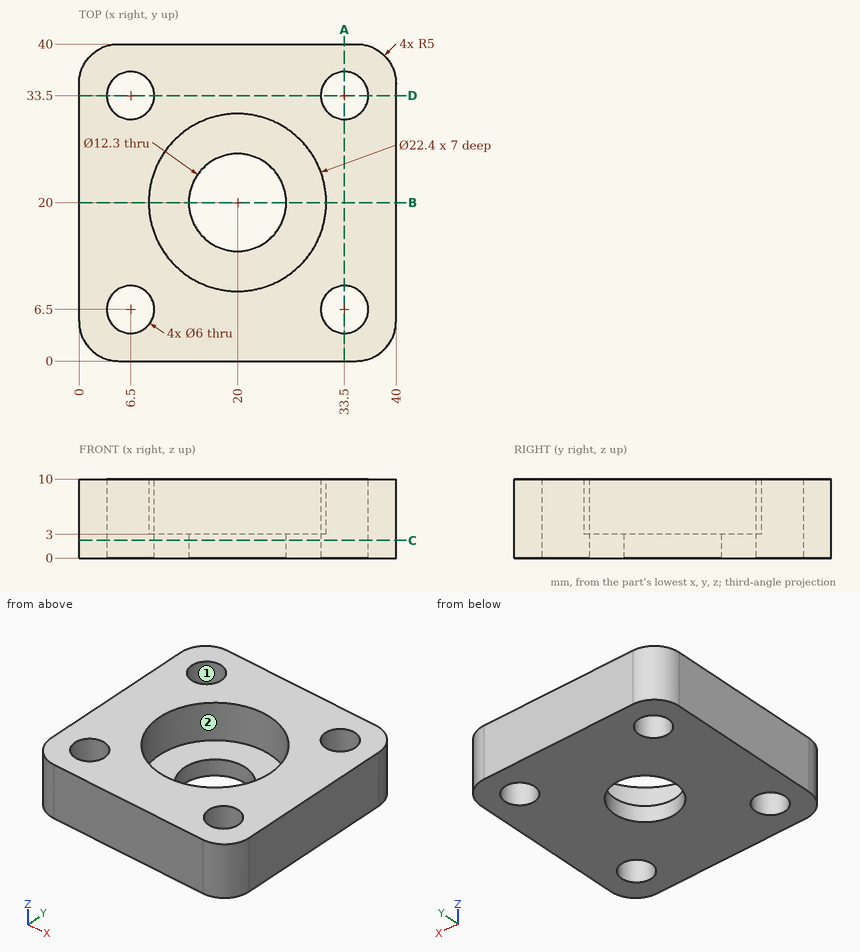
Drawing for the job (mm, zero at the part's lowest x, y, z). A direction names the side the tool comes from. Give positions to 0.01 mm unless a question says otherwise; leave off trailing zeros. Order: outer loops, then holes, each group sorted by start corner. A loop starts at its lowest first (then second) coordinate and runs counter-clockwise, first axis right, second up. Notation, with made-up numbers: (-5.5, 41.5) - (27.5, 41.5) arc R18 cw to (27.5, 60.5) - close; hole circle Ø5 at (-28.5, 60). An arc over 180 degrees is marked (long way). Write item = value, one per line. Start each with the question number.
1. Cut at A-A, the plane x = 33.5. List the corners of the cut face in (y, z), and give its area (3 significant figures).
2. Drop flat-ended pins along their axis: P1, Ø11, axis at x = 22.5, y = 15, coming from the +Z side; P2, Ø1, axis at x = 4, z = 5, coming from the +Y side. Give the stop position or say it passes through.
3. Cut at C-C, the plane z = 2.25. List the corners of the cut face in (x, y).
4. Which spindle directions (+Z, -Z, +X, -X, +Y, -Y) get a long thin tool onto all of the face, cutting with end or side? Do the marked faces 1 and 2. Say none if no direction does.
5. Cut at B-B, the plane y = 20. List the corners of the cut face in (x, z).
6. Probe line 1 along Y through (x, z) = (33.5, 4.25); line 2 along Y through (x, z) = (4, 6); line 3 along Y through (x, z) = (20, 1.05). List the from-to ranges inside material, lowest first.
Taken from the geometry:
q1.outline = (0, 0) - (3.5, 0) - (3.5, 10) - (0, 10) - close; (9.5, 0) - (30.5, 0) - (30.5, 10) - (9.5, 10) - close; (36.5, 0) - (40, 0) - (40, 10) - (36.5, 10) - close
q1.area = 280 mm²
q2.P1 = 3
q2.P2 = 39.97
q3.outline = (0, 5) arc R5 ccw to (5, 0) - (35, 0) arc R5 ccw to (40, 5) - (40, 35) arc R5 ccw to (35, 40) - (5, 40) arc R5 ccw to (0, 35) - close; hole circle Ø6 at (6.5, 6.5); hole circle Ø6 at (6.5, 33.5); hole circle Ø12.3 at (20, 20); hole circle Ø6 at (33.5, 6.5); hole circle Ø6 at (33.5, 33.5)
q4.face_1 = +Z, -Z
q4.face_2 = +Z
q5.outline = (0, 0) - (13.85, 0) - (13.85, 3) - (8.8, 3) - (8.8, 10) - (0, 10) - close; (26.15, 0) - (40, 0) - (40, 10) - (31.2, 10) - (31.2, 3) - (26.15, 3) - close
q6.line_1 = 0 to 3.5, 9.5 to 30.5, 36.5 to 40
q6.line_2 = 0.1 to 4.84, 8.16 to 31.84, 35.16 to 39.9
q6.line_3 = 0 to 13.85, 26.15 to 40
